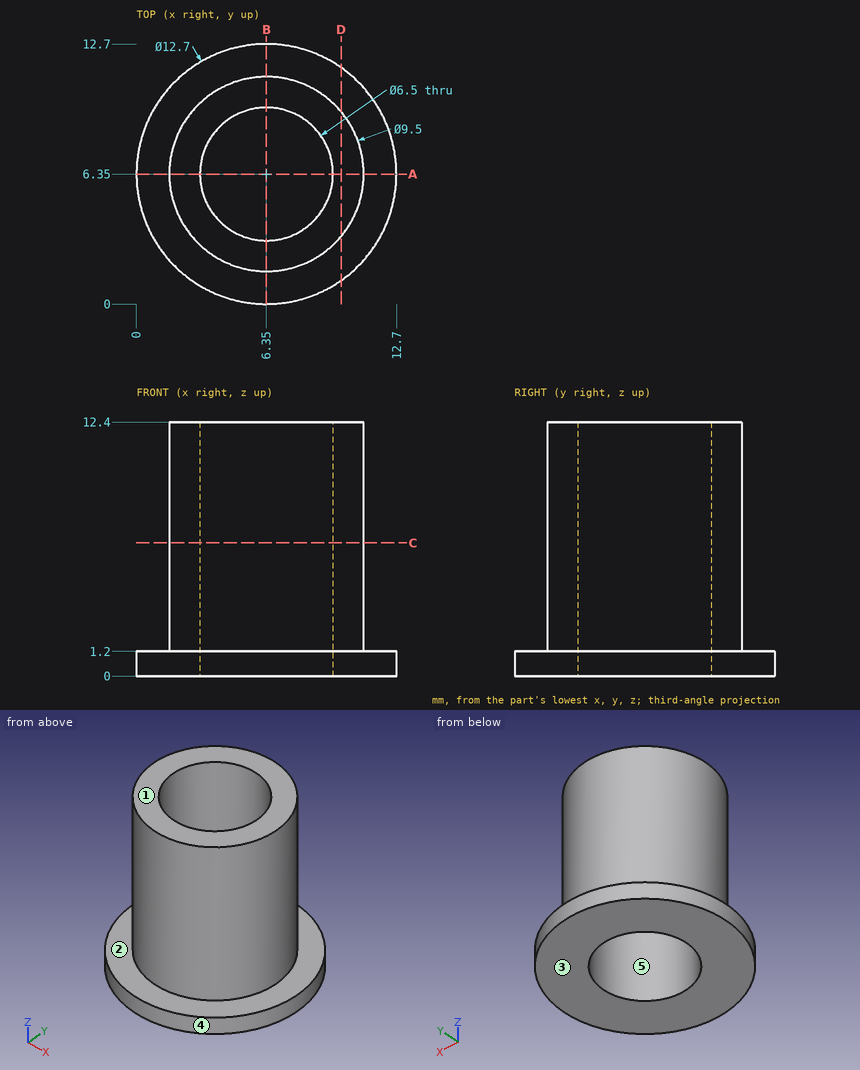
Check sheet for the drawn part. Datum: minimum x, y, z corner. Units: mm. A direction names the side the tool comes from. Coordinates: 2 decimals unless noted, no trailing zeros. Loops run counter-clockwise (first coordinate to the right, second up) from the corner with the lowest first, then second, coordinate; pieces in that order, holes last. Notation, with made-up numbers: (81.5, 41.25) -> (115.5, 41.25) arc R33 cw to (115.5, 80.25) -> close; hole circle Ø5 at (83, 13). An arc over 180 degrees is marked (long way). Answer in a Markdown table with one row per item.
1) Section check D-D (x = 10). Record the cut outline in (y, z).
The answers:
| item | result |
|---|---|
| outline | (1.15, 0) -> (11.55, 0) -> (11.55, 1.2) -> (9.39, 1.2) -> (9.39, 12.4) -> (3.31, 12.4) -> (3.31, 1.2) -> (1.15, 1.2) -> close |
2) Access from +Z, -Z, +X, -X, +Y, -Y to the whole of each face (thin tool, end or side, straight path). Record for the marked faces 1 and 2.
The answers:
| item | result |
|---|---|
| face 1 | +Z, +X, -X, +Y, -Y |
| face 2 | +Z |
3) Depth check by flat-ended pin: P1, Ø3, axis at x = 5.5, z = 5.5, coming from the +Y side; P2, Ø5, axis at y = 9, z = 1.5, coming from the +X side; P3, Ø1, axis at y = 2.5, z = 6.5, coming from the +X side. Enter the tip coordinate at first touch or a pass-through.
The answers:
| item | result |
|---|---|
| P1 | stops at y = 11.1 |
| P2 | stops at x = 12.7 |
| P3 | stops at x = 9.72 |
4) Section check A-A (y = 6.35). Record the cut outline in (x, z).
The answers:
| item | result |
|---|---|
| outline | (0, 0) -> (3.1, 0) -> (3.1, 12.4) -> (1.6, 12.4) -> (1.6, 1.2) -> (0, 1.2) -> close; (9.6, 0) -> (12.7, 0) -> (12.7, 1.2) -> (11.1, 1.2) -> (11.1, 12.4) -> (9.6, 12.4) -> close |
5) Scan lines: line 1 along Y through (x, z) = (6.25, 10.25); line 2 along Z through (x, y) = (1, 8.25); line 3 along Y through (x, z) = (5.5, 7.25). Record each from-to range of solid material in increasing order. Write a range as from..to.
The answers:
| item | result |
|---|---|
| line 1 | y = 1.6..3.1, 9.6..11.1 |
| line 2 | z = 0..1.2 |
| line 3 | y = 1.68..3.21, 9.49..11.02 |
6) Draft check along X on the marked faces 3, 4 and 5. Enter one of: released by +X, released by -X, zero draft, split by the parting line, or undercut.
The answers:
| item | result |
|---|---|
| face 3 | zero draft |
| face 4 | split by the parting line |
| face 5 | undercut |
7) Section check C-C (z = 6.5). Record the cut outline in (x, y), and give its area (3 significant figures).
The answers:
| item | result |
|---|---|
| outline | circle Ø9.5 at (6.35, 6.35); hole circle Ø6.5 at (6.35, 6.35) |
| area | 37.7 mm2 |
